from build123d import *

# Parameters (mm, degrees)
SKETCH1_W           = 40
SKETCH1_H           = 10
BOSS_EXTRUDE1_DEPTH = 5
SKETCH2_R           = 1
CUT_EXTRUDE1_DEPTH  = 5
FILLET1_R           = 5


with BuildPart() as part:
    # Sketch1 → Boss-Extrude1 (new body)
    with BuildSketch(Plane(origin=(0, 0, 0), x_dir=(1, 0, 0), z_dir=(0, 1, 0))):
        Rectangle(SKETCH1_W, SKETCH1_H)
    extrude(amount=BOSS_EXTRUDE1_DEPTH)

    # Sketch2 → Cut-Extrude1 (cut)
    with BuildSketch(Plane(origin=(0, 0, 0), x_dir=(1, 0, 0), z_dir=(0, 1, 0))):
        with Locations(Location((10, 0, 0), (0, 0, 270))):
            Circle(SKETCH2_R)
        with Locations(Location((15, 0, 0), (0, 0, 270))):
            Circle(SKETCH2_R)
        with Locations(Location((-10, 0, 0), (0, 0, 270))):
            Circle(SKETCH2_R)
        with Locations(Location((-14, 0, 0), (0, 0, 270))):
            Circle(SKETCH2_R)
    extrude(amount=CUT_EXTRUDE1_DEPTH, mode=Mode.SUBTRACT)

    # Fillet1
    fillet1_edges = [part.edges().sort_by_distance(p)[0] for p in [
        (20, 2.5, -5),
        (-20, 2.5, -5),
        (20, 2.5, 5),
        (-20, 2.5, 5),
    ]]
    fillet(fillet1_edges, radius=FILLET1_R - 0.0001)  # a hair under: the kernel refuses the full size


solid = part.part
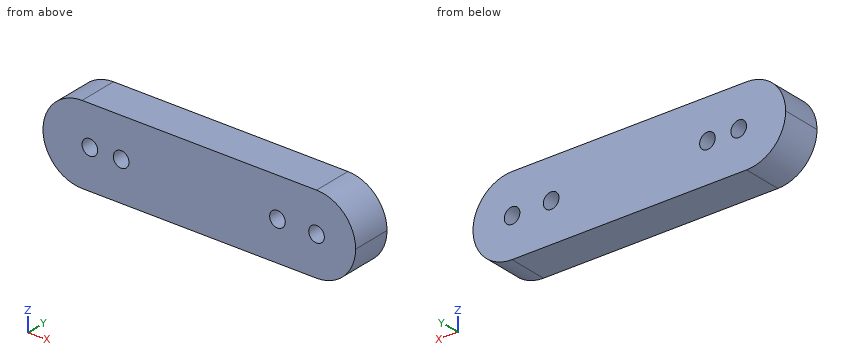
Can you work these out from the model? Positions are in its coordinate system, mm. Give positions to 0.01 mm unless a question says otherwise; leave off trailing zeros. Loops run counter-clockwise (first coordinate to the right, second up) from the corner with the lowest first, then second, coordinate; pieces in that order, holes last. Notation, with made-up numbers: (83.25, -19) - (138.25, -19) arc R23 ccw to (138.25, -2) - close; hole circle Ø10 at (88.5, 64). An arc over 180 degrees is marked (long way). Answer as a JSON object with one key per item and string values.
Q1. Imagine slicing it at B-B on y = 2.5. Give the number of separate pieces and of enclosed holes in the cut face, plus the area to 3 significant figures.
Geometry says:
{"separate pieces": "1", "enclosed holes": "4", "area": "366 mm²"}
Q2. Imagine slicing it at A-A on x = -14. Write out the boundary of the cut face in (y, z).
Geometry says:
{"outline": "(0, -5) - (5, -5) - (5, -1) - (0, -1) - close; (0, 1) - (5, 1) - (5, 5) - (0, 5) - close"}
Q3. Will this pin go through, and if not, where does the flat tip stop? P1, Ø2.5, axis at x = 10, z = 0, coming from the +Y side.
Geometry says:
{"P1": "y = 5"}
Q4. Imagine slicing it at C-C on x = 15.5. Write out the boundary of the cut face in (y, z).
Geometry says:
{"outline": "(0, -4.97) - (5, -4.97) - (5, -0.87) - (0, -0.87) - close; (0, 0.87) - (5, 0.87) - (5, 4.97) - (0, 4.97) - close"}
Q5. If I drill on L1, parallel to X at y = 2.05, z = 0; L2, parallel to X at y = 0.5, z = -0.5; L3, parallel to Z at x = -13.5, y = 1.55, over which ranges is the centre line in solid material (lowest first)?
Geometry says:
{"L1": "-20 to -15, -13 to -11, -9 to 9, 11 to 14, 16 to 20", "L2": "-19.97 to -14.87, -13.13 to -10.87, -9.13 to 9.13, 10.87 to 14.13, 15.87 to 19.97", "L3": "-5 to -0.87, 0.87 to 5"}
Q6. Imagine slicing it at D-D on z = -2.25. Write out the boundary of the cut face in (x, y).
Geometry says:
{"outline": "(-19.47, 0) - (19.47, 0) - (19.47, 5) - (-19.47, 5) - close"}
